Verification items for the finished model (mm, model axes). A direction names the side the tool comes from. Coordinates: 2 decimals unless noted, no trailing zeros. Loops run counter-clockwise (first coordinate to the right, second up) from the corner with the lowest first, then second, coordinate; pieces in that order, holes last. Notation, with made-up numbers: (77, 26.25) -> (131, 26.25) arc R20 ccw to (131, 52.25) -> close; hole circle Ø9 at (35.5, 69). An arc over 180 degrees is marked (long way). Write item = value, one per line.
```python
from build123d import *

# Parameters (mm, degrees)
CYLINDER043_R          = 2
CYLINDER043_DEPTH      = 10
CYLINDER044_R          = 2
CYLINDER044_DEPTH      = 10
CYLINDER042_R          = 2
CYLINDER042_DEPTH      = 10
CYLINDER041_R          = 2
CYLINDER041_DEPTH      = 10
CYLINDER040_R          = 4
CYLINDER040_DEPTH      = 60
CYLINDER045_R          = 7.5
CYLINDER045_DEPTH      = 40
BOX008_W               = 25
BOX008_H               = 25
BOX008_DEPTH           = 5.2
CUT038_ROLL_ANGLE      = -90
CUT038_PLACEMENT_ANGLE = -90


with BuildPart() as cylinder043:
    # Cylinder043 → Cylinder043 (new body)
    with BuildSketch(Plane(origin=(21, 21, -2), x_dir=(1, 0, 0), z_dir=(0, 0, 1))):
        Circle(CYLINDER043_R)
    extrude(amount=CYLINDER043_DEPTH)


with BuildPart() as cylinder044:
    # Cylinder044 → Cylinder044 (new body)
    with BuildSketch(Plane(origin=(21, 4, -2), x_dir=(1, 0, 0), z_dir=(0, 0, 1))):
        Circle(CYLINDER044_R)
    extrude(amount=CYLINDER044_DEPTH)


with BuildPart() as cylinder042:
    # Cylinder042 → Cylinder042 (new body)
    with BuildSketch(Plane(origin=(4, 21, -2), x_dir=(1, 0, 0), z_dir=(0, 0, 1))):
        Circle(CYLINDER042_R)
    extrude(amount=CYLINDER042_DEPTH)


with BuildPart() as cylinder041:
    # Cylinder041 → Cylinder041 (new body)
    with BuildSketch(Plane(origin=(4, 4, -2), x_dir=(1, 0, 0), z_dir=(0, 0, 1))):
        Circle(CYLINDER041_R)
    extrude(amount=CYLINDER041_DEPTH)


with BuildPart() as cylinder040:
    # Cylinder040 → Cylinder040 (new body)
    with BuildSketch(Plane(origin=(12.5, 12.5, -7), x_dir=(1, 0, 0), z_dir=(0, 0, 1))):
        Circle(CYLINDER040_R)
    extrude(amount=CYLINDER040_DEPTH)


with BuildPart() as cylinder045:
    # Cylinder045 → Cylinder045 (new body)
    with BuildSketch(Plane(origin=(12.5, 12.5, 5), x_dir=(1, 0, 0), z_dir=(0, 0, 1))):
        Circle(CYLINDER045_R)
    extrude(amount=CYLINDER045_DEPTH)


with BuildPart() as cut038:
    # Box008 → Box008 (new body)
    with BuildSketch(Plane.XY):
        with Locations((12.5, 12.5)):
            Rectangle(BOX008_W, BOX008_H)
    extrude(amount=BOX008_DEPTH)

    # Fusion009: union Cylinder045
    add(cylinder045.part)

    # Cut037: cut Cylinder040
    add(cylinder040.part, mode=Mode.SUBTRACT)

    # Cut036: cut Cylinder041
    add(cylinder041.part, mode=Mode.SUBTRACT)

    # Cut035: cut Cylinder042
    add(cylinder042.part, mode=Mode.SUBTRACT)

    # Cut034: cut Cylinder044
    add(cylinder044.part, mode=Mode.SUBTRACT)

    # Cut038: cut Cylinder043
    add(cylinder043.part, mode=Mode.SUBTRACT)


with BuildPart() as cut038_1:
    # Cut038 roll: moved
    add(cut038.part.rotate(Axis((0, 0, 0), (1, 0, 0)), CUT038_ROLL_ANGLE))


with BuildPart() as cut038_2:
    # Cut038 placement: moved
    add(cut038_1.part.moved(Location((94, 37.5, 72.5))).rotate(Axis((94, 37.5, 72.5), (0, 0, 1)), CUT038_PLACEMENT_ANGLE))


solid = cut038_2.part
```
1) Material ranges on line 1 (Z direction, x = 98.05, y = 16.5); line 2 (Z direction, x = 114, y = 25); line 3 (X direction, y = 18.5, z = 53.5), recorded low to high.
Ans:
line_1 = 47.5 to 49.5, 53.5 to 66.5, 70.5 to 72.5
line_2 = 52.5 to 56, 64 to 67.5
line_3 = 94 to 99.2
2) Sectioned sample at A-A, the plane z = 51.5. Record the cut outline in (x, y), plus the area to 3 significant figures.
Ans:
outline = (94, 12.5) -> (99.2, 12.5) -> (99.2, 14.5) -> (94, 14.5) -> close; (94, 18.5) -> (99.2, 18.5) -> (99.2, 31.5) -> (94, 31.5) -> close; (94, 35.5) -> (99.2, 35.5) -> (99.2, 37.5) -> (94, 37.5) -> close
area = 88.4 mm2
3) Depth check by flat-ended pin: pin 1 Ø5 at (x, z) = (126, 66.5) entering from -Y; pin 2 Ø8 at (y, z) = (20.5, 53) entering from +X; pin 3 Ø4 at (x, y) = (133.5, 31) entering from -Z; pin 4 Ø2 at (x, z) = (133, 53.5) entering from -Y. Enter the tip coordinate at first touch or a pass-through.
Ans:
pin_1 = 18.66
pin_2 = 139
pin_3 = 53.66
pin_4 = 19.9
4) Sectioned sample at B-B, the plane y = 33.5. Record the cut outline in (x, z).
Ans:
outline = (94, 47.5) -> (99.2, 47.5) -> (99.2, 49.5) -> (94, 49.5) -> close; (94, 53.5) -> (99.2, 53.5) -> (99.2, 66.5) -> (94, 66.5) -> close; (94, 70.5) -> (99.2, 70.5) -> (99.2, 72.5) -> (94, 72.5) -> close
5) Tool access check on faces 1 (the face through (97, 25, 47.5)), 2 (the face through (99.2, 31, 54)). Record the directions out of +Z, -Z, +X, -X, +Y, -Y that give a thin tool (end or side, any length) a straight path to the whole face; none if there is none.
Ans:
face_1 = -Z, +X, -X, +Y, -Y
face_2 = +X
6) Release check for a two-part mould opening along Y. For faces 3 (the face through (97, 12.5, 60)), 4 (the face through (94, 28, 57)), 5 (the face through (116.185, 25.867, 63.905)), 6 (the face through (96.564, 16.76, 66.517)) record: pulls with the +Y half, pulls with the -Y half, needs draft (parallel to the pull), parting line crosses it, or undercut.
Ans:
face_3 = pulls with the -Y half
face_4 = needs draft
face_5 = undercut
face_6 = undercut
7) Sectioned sample at D-D, the plane x = 131. Record the cut outline in (y, z), plus the area to 3 significant figures.
Ans:
outline = circle Ø15 at (25, 60); hole circle Ø8 at (25, 60)
area = 126 mm2
8) Sectioned sample at C-C, the plane y = 25. Record the cut outline in (x, z), plus the area to 3 significant figures.
Ans:
outline = (94, 47.5) -> (99.2, 47.5) -> (99.2, 52.5) -> (139, 52.5) -> (139, 56) -> (94, 56) -> close; (94, 64) -> (139, 64) -> (139, 67.5) -> (99.2, 67.5) -> (99.2, 72.5) -> (94, 72.5) -> close
area = 367 mm2
